```python
from build123d import *

# Parameters (mm, degrees)
SKETCH2_W           = 54.4
SKETCH2_H           = 16
BOSS_EXTRUDE1_DEPTH = 4
SKETCH3_W           = 2.3
SKETCH3_H           = 24
BOSS_EXTRUDE2_DEPTH = 54.4
SKETCH4_R           = 2.3
CUT_EXTRUDE1_DEPTH  = 45
CUT_EXTRUDE3_DEPTH  = 10
SKETCH5_R           = 8
CUT_EXTRUDE2_DEPTH  = 10
CUT_EXTRUDE4_DEPTH  = 10
SKETCH8_W           = 2.5
SKETCH8_H           = 10.25
BOSS_EXTRUDE3_DEPTH = 54.4
SKETCH9_W           = 2.5
SKETCH9_H           = 3.3
BOSS_EXTRUDE4_DEPTH = 10.25
CUT_EXTRUDE5_DEPTH  = 3.3
SKETCH11_W          = 54.4
SKETCH11_H          = 10.2
CUT_EXTRUDE6_DEPTH  = 10
BOSS_EXTRUDE5_DEPTH = 54.4
CUT_EXTRUDE7_DEPTH  = 54.4
SKETCH14_R          = 2.3
CUT_EXTRUDE8_DEPTH  = 54.4


with BuildPart() as part:
    # Sketch2 → Boss-Extrude1 (new body)
    with BuildSketch(Plane(origin=(0, 0, 0), x_dir=(1, 0, 0), z_dir=(0, 1, 0))):
        Rectangle(SKETCH2_W, SKETCH2_H)
    extrude(amount=BOSS_EXTRUDE1_DEPTH)

    # Sketch3 → Boss-Extrude2 (add)
    with BuildSketch(Plane(origin=(27.2, 0, 0), x_dir=(0, 0, -1), z_dir=(1, 0, 0))):
        with Locations((-9.15, 12)):
            Rectangle(SKETCH3_W, SKETCH3_H)
    extrude(amount=-BOSS_EXTRUDE2_DEPTH)

    # Sketch4 → Cut-Extrude1 (cut)
    with BuildSketch(Plane(origin=(0, 4, 0), x_dir=(1, 0, 0), z_dir=(0, 1, 0))):
        with Locations((-13.5, 2.5)):
            Circle(SKETCH4_R)
        with Locations((13.5, 2.5)):
            Circle(SKETCH4_R)
    extrude(amount=-CUT_EXTRUDE1_DEPTH, mode=Mode.SUBTRACT)

    # Sketch6 → Cut-Extrude3 (cut)
    with BuildSketch(Plane.XY.offset(10.3)):
        with BuildLine():
            Line((-3.75, 7.85), (3.75, 7.85))
            ThreePointArc((3.75, 7.85), (5.3, 6.3), (3.75, 4.75))
            Line((3.75, 4.75), (-3.75, 4.75))
            ThreePointArc((-3.75, 4.75), (-5.3, 6.3), (-3.75, 7.85))
        make_face()
    extrude(amount=-CUT_EXTRUDE3_DEPTH, mode=Mode.SUBTRACT)

    # Sketch5 → Cut-Extrude2 (cut)
    with BuildSketch(Plane.XY.offset(10.3)):
        with Locations((-13.5, 14.25)):
            Circle(SKETCH5_R)
        with Locations((13.5, 14.25)):
            Circle(SKETCH5_R)
    extrude(amount=-CUT_EXTRUDE2_DEPTH, mode=Mode.SUBTRACT)

    # Sketch7 → Cut-Extrude4 (cut)
    with BuildSketch(Plane.XY.offset(10.3)):
        Polygon((-35.24269893, 14.25), (-13.5, 14.25), (-5.3, 6.3), (0, 6.5), (5.3, 6.3), (13.5, 14.25), (21.5, 14.25), (36.006358293, 14.25), (36.006358293, 27.887641337), (-35.24269893, 27.887641337), align=None)
    extrude(amount=-CUT_EXTRUDE4_DEPTH, mode=Mode.SUBTRACT)

    # Sketch8 → Boss-Extrude3 (add)
    with BuildSketch(Plane(origin=(27.2, 0, 0), x_dir=(0, 0, -1), z_dir=(1, 0, 0))):
        with Locations((-3.45, 9.125)):
            Rectangle(SKETCH8_W, SKETCH8_H)
    extrude(amount=-BOSS_EXTRUDE3_DEPTH)

    # Sketch9 → Boss-Extrude4 (add)
    with BuildSketch(Plane(origin=(0, 4, 0), x_dir=(1, 0, 0), z_dir=(0, 1, 0))):
        with Locations((-25.95, -6.35)):
            Rectangle(SKETCH9_W, SKETCH9_H)
        with Locations((25.95, -6.35)):
            Rectangle(SKETCH9_W, SKETCH9_H)
    extrude(amount=BOSS_EXTRUDE4_DEPTH)

    # Sketch10 → Cut-Extrude5 (cut)
    with BuildSketch(Plane.XY.offset(4.7)):
        Polygon((-27.2, 8.25), (-25.2, 8.25), (-27.2, 11.25), align=None)
        Polygon((27.2, 11.25), (27.2, 8.25), (25.2, 8.25), align=None)
    extrude(amount=CUT_EXTRUDE5_DEPTH, mode=Mode.SUBTRACT)

    # Sketch11 → Cut-Extrude6 (cut)
    with BuildSketch(Plane(origin=(0, 4, 0), x_dir=(1, 0, 0), z_dir=(0, 1, 0))):
        with Locations((0, 2.9)):
            Rectangle(SKETCH11_W, SKETCH11_H)
    extrude(amount=-CUT_EXTRUDE6_DEPTH, mode=Mode.SUBTRACT)

    # Sketch12 → Boss-Extrude5 (add)
    with BuildSketch(Plane.ZY.offset(27.2)):
        Polygon((10.3, 0), (-7.522416627, 1.87321147), (-7.110333074, 5.793924586), (10.3, 3.964024842), align=None)
    extrude(amount=-BOSS_EXTRUDE5_DEPTH)

    # Sketch13 → Cut-Extrude7 (cut)
    with BuildSketch(Plane(origin=(27.2, 0, 0), x_dir=(0, 0, -1), z_dir=(1, 0, 0))):
        Polygon((-2.2, 0.851344306), (-10.3, 0), (-2.2, 0), align=None)
    extrude(amount=-CUT_EXTRUDE7_DEPTH, mode=Mode.SUBTRACT)

    # Sketch14 → Cut-Extrude8 (cut)
    with BuildSketch(Plane(origin=(0, 4.991458323, 0.52462341), x_dir=(1, 0, 0), z_dir=(0, 0.994521895, 0.104528463))):
        with Locations((-13.5, 2.904418591)):
            Circle(SKETCH14_R)
        with Locations((13.5, 2.904418591)):
            Circle(SKETCH14_R)
    extrude(amount=-CUT_EXTRUDE8_DEPTH, mode=Mode.SUBTRACT)


solid = part.part
```
Input: part model. Units: mm. Frame: model coordinates. A direction names the side the tool comes from. Give positions to 0.01 mm unless a question says otherwise; leave off trailing zeros. Order: outer loops, then holes, each group sorted by start corner. A loop starts at its lowest first (then second) coordinate and runs counter-clockwise, first axis right, second up. Notation, with made-up numbers: M 25.25,21 L 83.25,21 A36 ccw 83.25,59 Z; hole C 27.5,75.25 d2. An arc over 180 degrees is marked long. One line per question, with ' | ' between items.
1) Section A-A on x = 2. Output: boundary loops of the cut face in (y, z).
Filled in:
outline: M 0,10.3 L 1.87,-7.52 L 5.79,-7.11 L 4.82,2.2 L 14.25,2.2 L 14.25,4.7 L 4.55,4.7 L 4.21,8 L 4.75,8 L 4.75,10.3 Z
2) Section B-B on y = 7.5. Output: boundary loops of the cut face in (x, z).
Filled in:
outline: M -27.2,2.2 L 27.2,2.2 L 27.2,10.3 L 17.79,10.3 L 17.79,8 L 24.7,8 L 24.7,4.7 L -24.7,4.7 L -24.7,8 L -17.79,8 L -17.79,10.3 L -27.2,10.3 Z; M -9.21,8 L -6.54,8 L -6.54,10.3 L -9.21,10.3 Z; M 6.54,8 L 9.21,8 L 9.21,10.3 L 6.54,10.3 Z
3) Draft query along X for faces 1 (the face through (-16.627, 6.886, 9.166)), 2 (the face through (-27, 9, 4.7)). Return one class per face: pulls with the +X half, pulls with the -X half, needs draft (parallel to the pull), parting line crosses it, or undercut.
Filled in:
face 1: undercut | face 2: needs draft
4) Ray query, L1, parallel to Z at x = -21.5, y = 12.5; L2, parallel to X at y = 2.75, z = -1.5; L3, parallel to Z at x = -4, y = 12. Return the intervals inside material, ascending.
Filled in:
L1: z = 2.2 to 4.7, 8 to 10.3 | L2: x = -27.2 to -15.51, -11.49 to 11.49, 15.51 to 27.2 | L3: z = 2.2 to 4.7
5) Section D-D on z = 5.25. Output: boundary loops of the cut face in (x, y).
Filled in:
outline: M -27.2,0.53 L 27.2,0.53 L 27.2,8.25 L 25.2,8.25 L 27.2,11.25 L 27.2,14.25 L 24.7,14.25 L 24.7,4.49 L -24.7,4.49 L -24.7,14.25 L -27.2,14.25 L -27.2,11.25 L -25.2,8.25 L -27.2,8.25 Z
6) Section C-C on x = 13.5. Output: boundary loops of the cut face in (y, z), and give its area (3 significant figures).
Filled in:
outline: M 0,10.3 L 1.13,-0.49 L 5.05,-0.08 L 4.82,2.2 L 14.25,2.2 L 14.25,4.7 L 4.55,4.7 L 4.21,8 L 6.25,8 L 6.25,10.3 Z; M 1.61,-5.06 L 1.87,-7.52 L 5.79,-7.11 L 5.54,-4.65 Z | area: 80.6 mm2
7) Access query for faces 3 (the face through (-0.35, 4.38, 6.33)), 4 (the face through (-0.38, 5.31, -2.52)), 5 (the face through (27, 9, 8)), 6 (the face through (0, 4.75, 9)). Directions: +Z, -Z, +X, -X, +Y, -Y. A direction counts if a zero-diameter tool reaches every point of the face in a straight line with its end or side. Return the directions, or none.
Filled in:
face 3: +Y | face 4: +X, -X, +Y | face 5: +X | face 6: +Z, +Y
8) Contact query for flat-ended pins moving along their axis: P1, Ø4, axis at x = 3.5, z = 8, coming from the -Y side; P2, Ø1, axis at x = 26, y = 10.5, coming from the -Z side; P3, Ø1.5, axis at x = 13.5, y = 7.5, coming from the +Z side. Output: stop coordinate, or through.
Filled in:
P1: stops at y = 0.03 | P2: stops at z = 2.2 | P3: stops at z = 4.7
